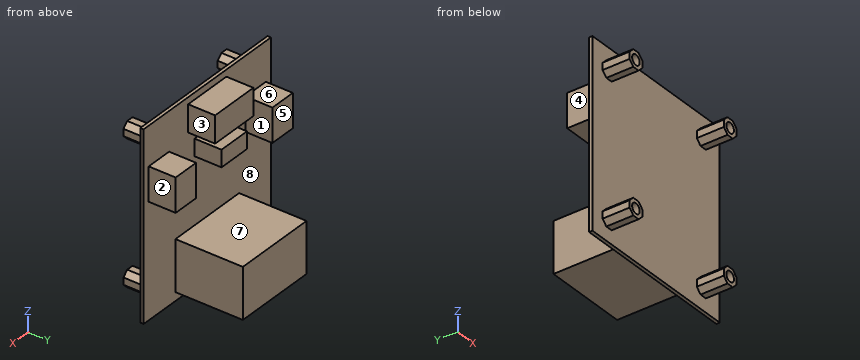
Autodesk Inventor part; units mm, degrees
ref_plane "YZ Plane" through (0, 0, 0) normal (1, 0, 0) x (0, 1, 0)
ref_plane "XZ Plane" through (0, 0, 0) normal (0, 1, 0) x (-1, 0, 0)
ref_plane "XY Plane" through (0, 0, 0) normal (0, 0, 1) x (1, 0, 0)
sketch "Esquisse1" plane through (0, 0, 0) normal (0, 1, 0) x (-1, 0, 0)
  line L0 (-25, 27.5) -> (25, 27.5)
  line L1 (25, 27.5) -> (25, -27.5)
  line L2 (25, -27.5) -> (-25, -27.5)
  line L3 (-25, -27.5) -> (-25, 27.5)
  point P0 (0, 0)
  dimension "d0" = 55
  dimension "d1" = 50
  dimension "d2" = 25
  dimension "d3" = 27.5
extrude "Extrusion1" add sketch "Esquisse1" along normal blind 1
sketch "Esquisse2" plane through (0, 1, 0) normal (0, 1, 0) x (1, 0, 0)
  line L0 (25, 27.5) -> (-25, 27.5)
  line L1 (-12.5, 25) -> (12.5, 25)
  line L2 (12.5, 25) -> (12.5, 10)
  line L3 (12.5, 10) -> (-12.5, 10)
  line L4 (-12.5, 10) -> (-12.5, 25)
  point P0 (0, 0)
  dimension "d6" = 15
  dimension "d7" = 25
  dimension "d8" = 12.5
  dimension "d9" = 2.5
extrude "Extrusion2" add sketch "Esquisse2" along normal blind 20
sketch "Esquisse3" plane through (0, 1, 0) normal (0, 1, 0) x (1, 0, 0)
  line L0 (-25, -27.5) -> (25, -27.5)
  line L1 (25, -27.5) -> (25, 27.5)
  line L2 (-25, 27.5) -> (-25, -27.5)
  line L3 (-23, -6) -> (-15, -6)
  line L4 (-15, -6) -> (-15, -16)
  line L5 (-15, -16) -> (-23, -16)
  line L6 (-23, -16) -> (-23, -6)
  line L7 (15, -6) -> (23, -6)
  line L8 (23, -6) -> (23, -16)
  line L9 (23, -16) -> (15, -16)
  line L10 (15, -16) -> (15, -6)
  line L11 (-7.5, -17.5) -> (7.5, -17.5)
  line L12 (7.5, -17.5) -> (7.5, -25.5)
  line L13 (7.5, -25.5) -> (-7.5, -25.5)
  line L14 (-7.5, -25.5) -> (-7.5, -17.5)
  line L15 (-5, -9.5) -> (5, -9.5)
  line L16 (5, -9.5) -> (5, -14.5)
  line L17 (5, -14.5) -> (-5, -14.5)
  line L18 (-5, -14.5) -> (-5, -9.5)
  point P0 (0, 0)
  dimension "d12" = 10
  dimension "d13" = 10
  dimension "d14" = 10
  dimension "d15" = 8
  dimension "d16" = 8
  dimension "d17" = 15
  dimension "d18" = 8
  dimension "d19" = 5
  dimension "d20" = 5
  dimension "d21" = 2
  dimension "d22" = 2
  dimension "d23" = 2
  dimension "d24" = 7.5
  dimension "d25" = 6
  dimension "d26" = 3
extrude "Extrusion3" add sketch "Esquisse3" along normal blind 8
sketch "Esquisse4" plane through (0, 0, 0) normal (0, -1, 0) x (1, 0, 0)
  line L0 (25, 27.5) -> (-25, 27.5)
  line L1 (-25, 27.5) -> (-25, -27.5)
  line L2 (-19.5355, 23.5) -> (-17.4645, 23.5)
  line L3 (-17.4645, 23.5) -> (-17.4645, 18.5) construction
  line L4 (-17.4645, 18.5) -> (-19.5355, 18.5)
  line L5 (-19.5355, 18.5) -> (-19.5355, 23.5) construction
  line L6 (-21, 22.0355) -> (-16, 22.0355) construction
  line L7 (-16, 22.0355) -> (-16, 19.9645)
  line L8 (-16, 19.9645) -> (-21, 19.9645) construction
  line L9 (-21, 19.9645) -> (-21, 22.0355)
  line L10 (-21, 22.0355) -> (-19.5355, 23.5)
  line L11 (-17.4645, 23.5) -> (-16, 22.0355)
  line L12 (-16, 19.9645) -> (-17.4645, 18.5)
  line L13 (-19.5355, 18.5) -> (-21, 19.9645)
  line L14 (-19.5355, 22.0355) -> (-17.4645, 19.9645) construction
  line L15 (-17.4645, 22.0355) -> (-19.5355, 19.9645) construction
  circle A0 centre (-18.5, 21) radius 1.5
  line L16 (0, 0) -> (0, 27.5) construction
  line L17 (0, 0) -> (-25, 0) construction
  line L18 (19.5355, 23.5) -> (17.4645, 23.5)
  line L19 (17.4645, 23.5) -> (17.4645, 18.5) construction
  line L20 (17.4645, 18.5) -> (19.5355, 18.5)
  line L21 (19.5355, 18.5) -> (19.5355, 23.5) construction
  line L22 (21, 22.0355) -> (16, 22.0355) construction
  line L23 (16, 22.0355) -> (16, 19.9645)
  line L24 (16, 19.9645) -> (21, 19.9645) construction
  line L25 (21, 19.9645) -> (21, 22.0355)
  line L26 (21, 22.0355) -> (19.5355, 23.5)
  line L27 (17.4645, 23.5) -> (16, 22.0355)
  line L28 (16, 19.9645) -> (17.4645, 18.5)
  line L29 (19.5355, 18.5) -> (21, 19.9645)
  line L30 (19.5355, 22.0355) -> (17.4645, 19.9645) construction
  line L31 (17.4645, 22.0355) -> (19.5355, 19.9645) construction
  circle A1 centre (18.5, 21) radius 1.5
  line L32 (-19.5355, -23.5) -> (-17.4645, -23.5)
  line L33 (-17.4645, -23.5) -> (-17.4645, -18.5) construction
  line L34 (-17.4645, -18.5) -> (-19.5355, -18.5)
  line L35 (-19.5355, -18.5) -> (-19.5355, -23.5) construction
  line L36 (-21, -22.0355) -> (-16, -22.0355) construction
  line L37 (-16, -22.0355) -> (-16, -19.9645)
  line L38 (-16, -19.9645) -> (-21, -19.9645) construction
  line L39 (-21, -19.9645) -> (-21, -22.0355)
  line L40 (-21, -22.0355) -> (-19.5355, -23.5)
  line L41 (-17.4645, -23.5) -> (-16, -22.0355)
  line L42 (-16, -19.9645) -> (-17.4645, -18.5)
  line L43 (-19.5355, -18.5) -> (-21, -19.9645)
  line L44 (-19.5355, -22.0355) -> (-17.4645, -19.9645) construction
  line L45 (-17.4645, -22.0355) -> (-19.5355, -19.9645) construction
  circle A2 centre (-18.5, -21) radius 1.5
  line L46 (16, -19.9645) -> (17.4645, -18.5)
  line L47 (17.4645, -18.5) -> (19.5355, -18.5)
  line L48 (16, -22.0355) -> (16, -19.9645)
  line L49 (16, -19.9645) -> (21, -19.9645) construction
  line L50 (19.5355, -18.5) -> (21, -19.9645)
  line L51 (17.4645, -23.5) -> (17.4645, -18.5) construction
  line L52 (17.4645, -23.5) -> (16, -22.0355)
  line L53 (19.5355, -22.0355) -> (17.4645, -19.9645) construction
  line L54 (17.4645, -22.0355) -> (19.5355, -19.9645) construction
  circle A3 centre (18.5, -21) radius 1.5
  line L55 (21, -22.0355) -> (16, -22.0355) construction
  line L56 (21, -19.9645) -> (21, -22.0355)
  line L57 (19.5355, -18.5) -> (19.5355, -23.5) construction
  line L58 (19.5355, -23.5) -> (17.4645, -23.5)
  line L59 (21, -22.0355) -> (19.5355, -23.5)
  dimension "d29" = 5
  dimension "d30" = 5
  dimension "d31" = 4
  dimension "d32" = 4
  dimension "d35" = 3
extrude "Extrusion4" add sketch "Esquisse4" along normal blind 8
equation "\"d14\" = d13"
equation "\"d16\" = d15"
equation "\"d22\" = d21"
equation "\"d23\" = d21"
equation "\"d30\" = d29"
properties part number "carte_puissance"
Read the model definition and answer for the solid it produces. Units are mm, in the model's axes. Face numbers are marked on the shaded views. A direction names the side the tool comes from. Coordinates: 2 decimals unless noted, no trailing zeros. Order: outer loops, then holes, each group sorted by start corner. A loop starts at its lowest first (then second) coordinate and runs counter-clockwise, first axis right, second up. Notation, with made-up numbers: (84.5, 19) -> (105.5, 19) arc R34 cw to (105.5, 57) -> close; hole circle Ø10 at (4.25, -32.75). An arc over 180 degrees is marked (long way). Answer as a JSON object with one key per item and string values.
1) Each of these flat-tipped pins is pushed along its axis until it touches: pin 1 (2.5 mm diameter, centred on x = -2.5, z = 11, fed in from +Y); pin 2 (10 mm diameter, centred on y = -3.5, z = -15.5, fed in from -X); pin 3 (4 mm diameter, centred on y = 4.5, z = 9.5, fed in from -X); pin 4 (1 mm diameter, centred on y = -4, z = 21, fed in from +X). Where does it stop, or does it pass through?
Model answer:
{"pin 1": "stops at y = 9", "pin 2": "stops at x = -25", "pin 3": "stops at x = -23", "pin 4": "stops at x = 21"}
2) A cutting plane is placed at D-D, the plane y = 11.25. Determine the outline of the cut face in (x, z), plus the area to 3 significant figures.
Model answer:
{"outline": "(-12.5, -25) -> (12.5, -25) -> (12.5, -10) -> (-12.5, -10) -> close", "area": "375 mm²"}
3) The mould has two halves that part along Z. Classify the marked faces 5, 6, 7 and 8: released by +Z, released by -Z, zero draft, split by the parting line, or undercut.
Model answer:
{"face 5": "zero draft", "face 6": "released by +Z", "face 7": "undercut", "face 8": "undercut"}
4) A cutting plane is placed at C-C, the plane z = 21. Determine the outline of the cut face in (x, y), plus the area to 3 significant figures.
Model answer:
{"outline": "(-25, 0) -> (-21, 0) -> (-21, -8) -> (-20, -8) -> (-20, 0) -> (-17, 0) -> (-17, -8) -> (-16, -8) -> (-16, 0) -> (16, 0) -> (16, -8) -> (17, -8) -> (17, 0) -> (20, 0) -> (20, -8) -> (21, -8) -> (21, 0) -> (25, 0) -> (25, 1) -> (7.5, 1) -> (7.5, 9) -> (-7.5, 9) -> (-7.5, 1) -> (-25, 1) -> close", "area": "202 mm²"}
5) A cutting plane is placed at A-A, the plane y = 7.5. Determine the outline of the cut face in (x, z).
Model answer:
{"outline": "(-23, 6) -> (-15, 6) -> (-15, 16) -> (-23, 16) -> close; (-12.5, -25) -> (12.5, -25) -> (12.5, -10) -> (-12.5, -10) -> close; (-7.5, 17.5) -> (7.5, 17.5) -> (7.5, 25.5) -> (-7.5, 25.5) -> close; (-5, 9.5) -> (5, 9.5) -> (5, 14.5) -> (-5, 14.5) -> close; (15, 6) -> (23, 6) -> (23, 16) -> (15, 16) -> close"}
6) A cutting plane is placed at B-B, the plane x = -1.5. Determine the outline of the cut face in (y, z), plus the area to 3 significant figures.
Model answer:
{"outline": "(0, -27.5) -> (1, -27.5) -> (1, -25) -> (21, -25) -> (21, -10) -> (1, -10) -> (1, 9.5) -> (9, 9.5) -> (9, 14.5) -> (1, 14.5) -> (1, 17.5) -> (9, 17.5) -> (9, 25.5) -> (1, 25.5) -> (1, 27.5) -> (0, 27.5) -> close", "area": "459 mm²"}
7) A tool of negligible diameter and unlimited length cuts with its end or side. For the marked faces 1, 2, 3 and 4, from which of +Z, -Z, +X, -X, +Y, -Y can it reach the whole face along a straight path? Write none if from no direction.
Model answer:
{"face 1": "+Z, -Z, +Y", "face 2": "+Z, -Z, +X, +Y", "face 3": "+Z, +X, +Y", "face 4": "+Z, -Z, -X, +Y"}
8) Consider line 1 along Z through (x, y) = (18.5, -1.75); line 2 along X through (y, z) = (20.25, -10.5); line 3 along Z through (x, y) = (-1, 18). Determine where each line is inside the solid, lowest interval first. Write a range as from..to.
Model answer:
{"line 1": "z = -23.5..-22.5, -19.5..-18.5, 18.5..19.5, 22.5..23.5", "line 2": "x = -12.5..12.5", "line 3": "z = -25..-10"}
